```python
from build123d import *

# Parameters (mm, degrees)
SKETCH1_R                       = 18.4277
BOSS_EXTRUDE1_DEPTH             = 29.5402
SKETCH2_R                       = 5.9563
BOSS_EXTRUDE2_DEPTH             = 4.953
SKETCH3_R                       = 3
BOSS_EXTRUDE3_DEPTH             = 15.2654
CUT_EXTRUDE1_DEPTH              = 13.8176
SKETCH5_R                       = 17.7419
BOSS_EXTRUDE4_DEPTH             = 33.2232
SKETCH6_R                       = 5.0292
BOSS_EXTRUDE5_DEPTH             = 3.048
CHAMFER1_SIZE                   = 1.5875
TAP_DRILL_FOR_M3X0_5_TAP1_D     = 2.5
TAP_DRILL_FOR_M3X0_5_TAP1_DEPTH = 5.08
TAP_DRILL_FOR_M3X0_5_TAP1_TIP   = 0.751075774


with BuildPart() as part:
    # Sketch1 → Boss-Extrude1 (new body)
    with BuildSketch(Plane(origin=(0, 0, 0), x_dir=(1, 0, 0), z_dir=(0, 1, 0))):
        with Locations(Location((0, 0, 0), (0, 0, 270))):
            Circle(SKETCH1_R)
    extrude(amount=BOSS_EXTRUDE1_DEPTH)

    # Sketch2 → Boss-Extrude2 (add)
    with BuildSketch(Plane(origin=(0, 29.5402, 0), x_dir=(1, 0, 0), z_dir=(0, 1, 0))):
        with Locations(Location((0, 0, 0), (0, 0, 270))):
            Circle(SKETCH2_R)
    extrude(amount=BOSS_EXTRUDE2_DEPTH)

    # Sketch3 → Boss-Extrude3 (add)
    with BuildSketch(Plane(origin=(0, 34.4932, 0), x_dir=(1, 0, 0), z_dir=(0, 1, 0))):
        with Locations(Location((0, 0, 0), (0, 0, 270))):
            Circle(SKETCH3_R)
    extrude(amount=BOSS_EXTRUDE3_DEPTH)

    # Sketch4 → Cut-Extrude1 (cut)
    with BuildSketch(Plane(origin=(0, 49.7586, 0), x_dir=(1, 0, 0), z_dir=(0, 1, 0))):
        with BuildLine():
            Line((-1.75155103, -2.435592791), (1.75155103, -2.435592791))
            ThreePointArc((1.75155103, -2.435592791), (0, -3.000007209), (-1.75155103, -2.435592791))
        make_face()
    extrude(amount=-CUT_EXTRUDE1_DEPTH, mode=Mode.SUBTRACT)

    # Sketch5 → Boss-Extrude4 (add)
    with BuildSketch(Plane.XZ):
        with Locations(Location((0, 0, 0), (0, 0, 270))):
            Circle(SKETCH5_R)
    extrude(amount=BOSS_EXTRUDE4_DEPTH)

    # Sketch6 → Boss-Extrude5 (add)
    with BuildSketch(Plane(origin=(0, -33.2232, 0), x_dir=(-1, 0, 0), z_dir=(0, -1, 0))):
        with Locations(Location((0, 0, 0), (0, 0, 90))):
            Circle(SKETCH6_R)
    extrude(amount=BOSS_EXTRUDE5_DEPTH)

    # Chamfer1
    chamfer1_edges = [part.edges().sort_by_distance(p)[0] for p in [
        (0, -36.2712, 5.0292),
    ]]
    chamfer(chamfer1_edges, length=CHAMFER1_SIZE)

    # Tap Drill for M3x0.5 Tap1
    with Locations(Plane(origin=(0, 29.5402, 0), x_dir=(1, 0, 0), z_dir=(0, 1, 0))):
        with Locations((0, 15.5), (13.423393759, 7.75), (13.423393759, -7.75), (0, -15.5), (-13.423393759, -7.75), (-13.423393759, 7.75)):
            Hole(TAP_DRILL_FOR_M3X0_5_TAP1_D / 2, depth=TAP_DRILL_FOR_M3X0_5_TAP1_DEPTH)
            with Locations((0, 0, -(TAP_DRILL_FOR_M3X0_5_TAP1_DEPTH + TAP_DRILL_FOR_M3X0_5_TAP1_TIP / 2))):  # 118° drill point
                Cone(0, TAP_DRILL_FOR_M3X0_5_TAP1_D / 2, TAP_DRILL_FOR_M3X0_5_TAP1_TIP, mode=Mode.SUBTRACT)


solid = part.part
```
Can you work these out from the model? Positions are in its coordinate system, mm. A direction names the side the tool comes from. Give positions to 0.01 mm unless a question says otherwise; leave off trailing zeros. Loops run counter-clockwise (first coordinate to the right, second up) from the corner with the lowest first, then second, coordinate; pieces in that order, holes last. Notation, with made-up numbers: M 61,22 L 95,22 A29 ccw 95,42 Z; hole C 7.25,-40 d10. An arc over 180 degrees is marked long. One line per item, written item: value.
(1) Suppose I cut it at C-C on z = 13. List the corners of the cut face in (x, y) for me, plus the area to 3 significant figures.
Returned:
outline: M -13.06,0 L -12.07,0 L -12.07,-33.22 L 12.07,-33.22 L 12.07,0 L 13.06,0 L 13.06,29.54 L -13.06,29.54 Z
area: 1,570 mm^2
(2) Suppose I cut it at D-D on y = -2. List the corners of the cut face in (x, z) for me, plus the area to 3 significant figures.
Returned:
outline: C 0,0 d35.48
area: 989 mm^2
(3) We'd pull the mould along X, two halves only. Please class faces 4 (the face through (12.27, 26.96, -7.27)), 5 (the face through (15, 0, -10)), 6 (the face through (0, 42, -3)): released by +X, released by -X, zero draft, split by the parting line, or undercut.
Returned:
face 4: undercut
face 5: zero draft
face 6: split by the parting line
(4) Will these pins go through, and if not, where does the flat tip stop? pin 1 (2 mm diameter, centred on x = 0, z = 15.5, fed in from -Y); pin 2 (10 mm diameter, centred on x = 12.5, y = 12.5, fed in from +Z); pin 3 (5 mm diameter, centred on x = 6.5, z = -3, fed in from +Y).
Returned:
pin 1: y = -33.22
pin 2: z = 16.83
pin 3: y = 34.49
(5) Suppose I cut it at B-B on y = 31.5. List the corners of the cut face in (x, z) for me.
Returned:
outline: C 0,0 d11.91
(6) Suppose I cut it at A-A on z = 0. List the corners of the cut face in (x, y) for me, plus the area to 3 significant figures.
Returned:
outline: M -18.43,0 L -17.74,0 L -17.74,-33.22 L -5.03,-33.22 L -5.03,-34.68 L -3.44,-36.27 L 3.44,-36.27 L 5.03,-34.68 L 5.03,-33.22 L 17.74,-33.22 L 17.74,0 L 18.43,0 L 18.43,29.54 L 5.96,29.54 L 5.96,34.49 L 3,34.49 L 3,49.76 L -3,49.76 L -3,34.49 L -5.96,34.49 L -5.96,29.54 L -18.43,29.54 Z
area: 2,450 mm^2
(7) I need wall thicknesses on line 1 (X direction, y = 25.95, z = 7.75); line 2 (Y direction, x = -14, z = -5); line 3 (X direction, y = 26.5, z = -15.5). Which ranges of each line are inside material? Lowest first, please.
Returned:
line 1: -16.72 to -14.67, -12.17 to 12.17, 14.67 to 16.72
line 2: -33.22 to 29.54
line 3: -9.97 to -1.25, 1.25 to 9.97
(8) Which directions (+Z, -Z, +X, -X, +Y, -Y) give clear straight access to the entire face, cutting with the end or side of a thin tool? Please do faces 1 (the face through (-12.43, 26.96, -6.99)), 2 (the face through (-4.91, -33.94, 1.09)), 3 (the face through (0, 43, 2.436)).
Returned:
face 1: +Y
face 2: -Y
face 3: +Z, +X, -X, +Y
